Autodesk Inventor part; units mm, degrees
ref_plane "YZ Plane" through (0, 0, 0) normal (1, 0, 0) x (0, 1, 0)
ref_plane "XZ Plane" through (0, 0, 0) normal (0, 1, 0) x (-1, 0, 0)
ref_plane "XY Plane" through (0, 0, 0) normal (0, 0, 1) x (1, 0, 0)
sketch "Sketch1" plane through (0, 0, 0) normal (0, 1, 0) x (-1, 0, 0)
  line L0 (-12.7, 15.875) -> (12.7, 15.875)
  line L1 (12.7, 15.875) -> (12.7, -15.875)
  line L2 (12.7, -15.875) -> (-12.7, -15.875)
  line L3 (-12.7, -15.875) -> (-12.7, 15.875)
  line L4 (-12.7, 15.875) -> (12.7, -15.875) construction
  line L5 (12.7, 15.875) -> (-12.7, -15.875) construction
  point P0 (0, 0)
  dimension "d0" = 25.4
  dimension "d1" = 31.75
extrude "Extrusion1" add sketch "Sketch1" along normal mid plane 3.175
sketch "Sketch2" plane through (0, 1.5875, 0) normal (0, 1, 0) x (1, 0, 0)
  line L0 (-12.7, 15.875) -> (-12.7, -15.875)
  line L1 (-12.7, -15.875) -> (-9.525, -15.875)
  line L2 (-9.525, -15.875) -> (-9.525, 15.875)
  line L3 (-9.525, 15.875) -> (-12.7, 15.875)
  line L4 (-12.7, 15.875) -> (-12.7, -15.875)
  line L5 (12.7, 15.875) -> (-12.7, 15.875)
  point P0 (0, 0)
  point P1 (-12.7, 15.875)
  dimension "d4" = 3.175
extrude "Extrusion2" add sketch "Sketch2" along normal blind 22.225
sketch "Sketch3" plane through (0, 1.5875, 0) normal (0, 1, 0) x (1, 0, 0)
  line L0 (-9.525, -15.875) -> (12.7, -15.875) construction
  line L1 (12.7, 15.875) -> (-9.525, 15.875) construction
  line L2 (-9.525, 15.875) -> (-9.525, -15.875) construction
  line L3 (-9.525, -15.875) -> (12.7, -15.875)
  line L4 (12.7, -15.875) -> (12.7, 15.875) construction
  line L5 (12.7, 15.875) -> (-9.525, 15.875)
  line L6 (1.5875, 15.875) -> (1.5875, -15.875) construction
  line L7 (12.7, -15.875) -> (-12.7, -15.875)
  line L8 (12.7, 0) -> (-9.525, 0) construction
  circle A0 centre (1.5875, 0) radius 7.5
  circle A1 centre (-5.4125, -12) radius 2
  circle A2 centre (-5.4125, 12) radius 2
  circle A3 centre (8.5875, -12) radius 2
  circle A4 centre (8.5875, 12) radius 2
  circle A5 centre (1.5875, 0) radius 8.5 construction
  circle A6 centre (-5.4125, -12) radius 3.5 construction
  point P0 (0, 0)
  dimension "d8" = 15
  dimension "d11" = 4
  dimension "d12" = 7
  dimension "d13" = 12
  dimension "d16" = 17
  dimension "d17" = 7
extrude "Extrusion3" cut sketch "Sketch3" against normal up to surface (3.175 mm away)
sketch "Sketch4" plane through (-9.525, 1.5875, 15.875) normal (1, 0, 0) x (0, 0, -1)
  line L0 (31.75, 0) -> (0, 0) construction
  line L1 (31.75, 0) -> (31.75, 22.225) construction
  line L2 (0, 22.225) -> (31.75, 22.225) construction
  line L3 (0, 0) -> (0, 22.225) construction
  line L4 (0, 11.1125) -> (31.75, 11.1125) construction
  line L5 (15.875, 22.225) -> (15.875, 0) construction
  circle A0 centre (15.875, 11.1125) radius 7.5
  circle A1 centre (3.875, 18.1125) radius 2
  circle A2 centre (3.875, 4.1125) radius 2
  circle A3 centre (27.875, 18.1125) radius 2
  circle A4 centre (27.875, 4.1125) radius 2
  point P0 (15.875, -1.5875)
  dimension "d18" = 15
  dimension "d19" = 4
  dimension "d20" = 12
  dimension "d21" = 7
extrude "Extrusion4" cut sketch "Sketch4" against normal up to surface (3.175 mm away)
chamfer "Chamfer1" distance 2 angle 45 4 edges at (12.7, 0, 15.875) (12.7, 0, -15.875) (-11.1125, 23.8125, -15.875) (-11.1125, 23.8125, 15.875)
properties part number "Custom L Bracket"
Here's how the part is built. I have some questions about the finished solid (model axes, mm). A direction names the side the tool comes from. Round coordinates to 2 decimals unless told otherwise and drop trailing zeros. Write each loop counter-clockwise with the first axis right and the second up, starting at its lowest first coordinate (ties: lowest second). Pieces come first, ordered by that corner, then holes.
Q1. If we mould it in two halves opening along Y, with no side actions, what happens to faces 1 (the flat face through (-6, 1, 15.875)), 2 (the flat face through (-11.13, 22.83, -14.86)), 3 (the cylindrical face through (-11.09, 7.052, -10.526))? For each: +Y half, -Y half, draft (parallel to the pull), parting line (faces both ways), or undercut.
Q2. If we section it at B-B on z = -12: Write out the boundary of the cut face in (x, y) (1 decimal).
Q3. If we section it at D-D on z = 0: Write out the boundary of the cut face in (x, y) (1 decimal), plus the area to 3 significant figures.
Q4. If we section it at C-C on x = 9.5: Write out the boundary of the cut face in (y, z) (1 decimal), plus the area to 3 significant figures.
Q5. Please list where these lines run through material, in increasing order: probe 1 along Y at (x, z) = (-10.5, -12); probe 2 along X at (y, z) = (-0.8, 12); probe 3 along X at (y, z) = (0.25, 0).
Q6. Which directions (+Z, -Z, +X, -X, +Y, -Y) give clear straight access to the entire face, cutting with the end or side of a thin tool? Please do faces 4 (the flat face through (-9.525, 10.1, 7.3)), 5 (the flat face through (-12.7, 5, -4)).
Q7. Will these pins go through, and if not, where does the flat tip stop? P1, Ø5, axis at x = 8.59, z = 12, coming from the +Y side; P2, Ø4, axis at y = 9.5, z = -11.5, coming from the +X side (3 decimals).
Q8. If we section it at A-A on y = 12.7: Write out the boundary of the cut face in (x, z) (3 decimals).
Answer below:
1. face 1: draft
1. face 2: +Y half
1. face 3: undercut
2. outline: (-12.7, -1.6) - (-7.4, -1.6) - (-7.4, 1.6) - (-9.5, 1.6) - (-9.5, 3.7) - (-12.7, 3.7) - close; (-12.7, 7.7) - (-9.5, 7.7) - (-9.5, 17.7) - (-12.7, 17.7) - close; (-12.7, 21.7) - (-9.5, 21.7) - (-9.5, 23.8) - (-12.7, 23.8) - close; (-3.4, -1.6) - (6.6, -1.6) - (6.6, 1.6) - (-3.4, 1.6) - close; (10.6, -1.6) - (12.7, -1.6) - (12.7, 1.6) - (10.6, 1.6) - close
3. outline: (-12.7, -1.6) - (-5.9, -1.6) - (-5.9, 1.6) - (-9.5, 1.6) - (-9.5, 5.2) - (-12.7, 5.2) - close; (-12.7, 20.2) - (-9.5, 20.2) - (-9.5, 23.8) - (-12.7, 23.8) - close; (9.1, -1.6) - (12.7, -1.6) - (12.7, 1.6) - (9.1, 1.6) - close
3. area: 56.0 mm2
4. outline: (-1.6, -15.9) - (1.6, -15.9) - (1.6, -13.8) - (-1.6, -13.8) - close; (-1.6, -10.2) - (1.6, -10.2) - (1.6, 10.2) - (-1.6, 10.2) - close; (-1.6, 13.8) - (1.6, 13.8) - (1.6, 15.9) - (-1.6, 15.9) - close
4. area: 78.2 mm2
5. probe 1: y = -1.59 to 3.7, 7.7 to 17.7, 21.7 to 23.81
5. probe 2: x = -12.7 to -7.41, -3.41 to 6.59, 10.59 to 12.7
5. probe 3: x = -12.7 to -5.91, 9.09 to 12.7
6. face 4: +Z, -Z, +X, +Y
6. face 5: +Z, -Z, -X, +Y, -Y
7. P1: stops at y = 1.59
7. P2: stops at x = -9.525
8. outline: (-12.7, -15.875) - (-9.525, -15.875) - (-9.525, -7.5) - (-12.7, -7.5) - close; (-12.7, 7.5) - (-9.525, 7.5) - (-9.525, 15.875) - (-12.7, 15.875) - close
